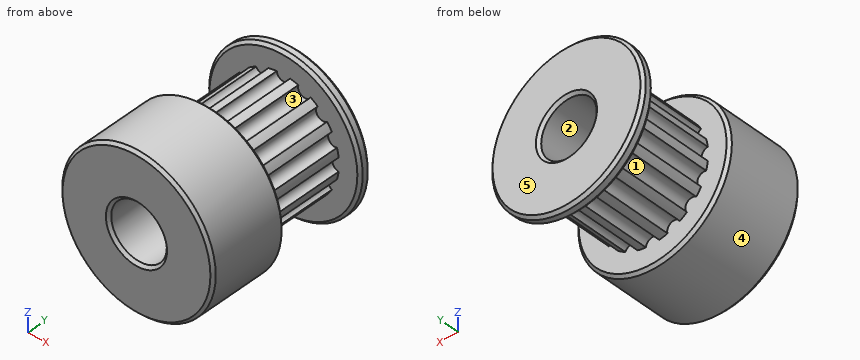
from build123d import *

# Parameters (mm, degrees)
F0_R     = 6.9
F1_DEPTH = 1
F2_R     = 5
F3_DEPTH = 7.5
F4_R     = 6.9
F5_DEPTH = 7
F6_R     = 0.6
F7_DEPTH = 7.5
F8_R     = 2.5
F9_DEPTH = 15.501
F10_SIZE = 0.25


with BuildPart() as f1:
    # F0 (on Front) → F1 (new body)
    with BuildSketch(Plane.XZ):
        Circle(F0_R)
    extrude(amount=F1_DEPTH)

    # F2 (on face) → F3 (join)
    with BuildSketch(Plane.XZ.offset(1)):
        Circle(F2_R)
    extrude(amount=F3_DEPTH)

    # F4 (on face) → F5 (join)
    with BuildSketch(Plane.XZ.offset(8.5)):
        Circle(F4_R)
    extrude(amount=F5_DEPTH)

    # F6 (on face) → F7 (cut, through all)
    with BuildSketch(Plane.XZ.offset(1)):
        with Locations((0, 5)):
            Circle(F6_R)
        with Locations((-1.913417, 4.619398)):
            Circle(F6_R)
        with Locations((-3.535534, 3.535534)):
            Circle(F6_R)
        with Locations((-4.619398, 1.913417)):
            Circle(F6_R)
        with Locations((-5, 0)):
            Circle(F6_R)
        with Locations((-4.619398, -1.913417)):
            Circle(F6_R)
        with Locations((-3.535534, -3.535534)):
            Circle(F6_R)
        with Locations((-1.913417, -4.619398)):
            Circle(F6_R)
        with Locations((0, -5)):
            Circle(F6_R)
        with Locations((1.913417, -4.619398)):
            Circle(F6_R)
        with Locations((3.535534, -3.535534)):
            Circle(F6_R)
        with Locations((4.619398, -1.913417)):
            Circle(F6_R)
        with Locations((5, 0)):
            Circle(F6_R)
        with Locations((4.619398, 1.913417)):
            Circle(F6_R)
        with Locations((3.535534, 3.535534)):
            Circle(F6_R)
        with Locations((1.913417, 4.619398)):
            Circle(F6_R)
    extrude(amount=F7_DEPTH, mode=Mode.SUBTRACT)

    # F8 (on face) → F9 (cut, through all)
    with BuildSketch(Plane.XZ.offset(15.5)):
        Circle(F8_R)
    extrude(amount=-F9_DEPTH, mode=Mode.SUBTRACT)

    # F10
    f10_edges = [f1.edges().sort_by_distance(p)[0] for p in [
        (6.9, -12, 0),
        (-6.9, -8.5, 0),
        (-6.9, -15.5, 0),
        (6.9, -0.5, 0),
        (-6.9, 0, 0),
        (-6.9, -1, 0),
        (-2.5, -15.5, 0),
        (2.5, -7.75, 0),
        (-2.5, 0, 0),
    ]]
    chamfer(f10_edges, length=F10_SIZE)


solid = f1.part
Verification items for the finished model (mm, model axes). Face numbers are marked on the shaded views. A direction names the side the tool comes from. Coordinates: 2 decimals unless noted, no trailing zeros. Loops run counter-clockwise (first coordinate to the right, second up) from the corner with the lowest first, then second, coordinate; pieces in that order, holes last. Notation, with made-up numbers: (36.25, -35) -> (93.25, -35) arc R24 cw to (93.25, -23) -> close; hole circle Ø9 at (69.5, 23). An arc over 180 degrees is marked (long way). Answer as CSV lines item,"result".
1) Depth check by flat-ended pin: pin 1 (5 mm diameter, centred on y = -12.5, z = -4, fed in from -X) (3 decimals); pin 2 (1.5 mm diameter, centred on y = -6.5, z = 5, fed in from -X); pin 3 (1.5 mm diameter, centred on x = 3.5, y = -4, fed in from +Z). Enter the tip coordinate at first touch or a pass-through.
Found:
pin 1,"stops at x = -6.735"
pin 2,"stops at x = -2.63"
pin 3,"stops at z = 4.18"
2) Cross-section at C-C, the plane z = 0. Record the cut outline in (x, y), then the cut area to 3 significant figures.
Found:
outline,"(-6.9, -15.25) -> (-6.65, -15.5) -> (-2.75, -15.5) -> (-2.5, -15.25) -> (-2.5, -0.25) -> (-2.75, 0) -> (-6.65, 0) -> (-6.9, -0.25) -> (-6.9, -0.75) -> (-6.65, -1) -> (-4.4, -1) -> (-4.4, -8.5) -> (-6.65, -8.5) -> (-6.9, -8.75) -> close; (2.5, -15.25) -> (2.75, -15.5) -> (6.65, -15.5) -> (6.9, -15.25) -> (6.9, -8.75) -> (6.65, -8.5) -> (4.4, -8.5) -> (4.4, -1) -> (6.65, -1) -> (6.9, -0.75) -> (6.9, -0.25) -> (6.65, 0) -> (2.75, 0) -> (2.5, -0.25) -> close"
area,"98.5 mm2"
3) Cross-section at A-A, the plane x = 0. Record the cut outline in (y, z).
Found:
outline,"(-15.5, -6.65) -> (-15.25, -6.9) -> (-8.75, -6.9) -> (-8.5, -6.65) -> (-8.5, -4.4) -> (-1, -4.4) -> (-1, -6.65) -> (-0.75, -6.9) -> (-0.25, -6.9) -> (0, -6.65) -> (0, -2.75) -> (-0.25, -2.5) -> (-15.25, -2.5) -> (-15.5, -2.75) -> close; (-15.5, 2.75) -> (-15.25, 2.5) -> (-0.25, 2.5) -> (0, 2.75) -> (0, 6.65) -> (-0.25, 6.9) -> (-0.75, 6.9) -> (-1, 6.65) -> (-1, 4.4) -> (-8.5, 4.4) -> (-8.5, 6.65) -> (-8.75, 6.9) -> (-15.25, 6.9) -> (-15.5, 6.65) -> close"
4) Cross-section at D-D, the plane y = -14.25. Record the cut outline in (x, z).
Found:
outline,"circle Ø13.8 at (0, 0); hole circle Ø5 at (0, 0)"
5) Tool access check on the marked faces 1 and 2. Record the directions out of +Z, -Z, +X, -X, +Y, -Y that give a thin tool (end or side, any length) a straight path to the whole face; none if there is none.
Found:
face 1,"none"
face 2,"+Y, -Y"
6) Thickness scan on L1, parallel to Y at x = 3, z = -4.25; L2, parallel to Z at x = 0, y = -7; L3, parallel to Z at x = -3, y = -3.25. Record the ranges inside material, lowest first. Write a range as from..to.
Found:
L1,"y = -15.5..-8.5, -1..0"
L2,"z = -4.4..-2.5, 2.5..4.4"
L3,"z = -4..-3.81, -3.26..3.26, 3.81..4"
7) Release check for a two-part mould opening along Z. For the marked faces 3, 4 and 5 record: +Z half, -Z half, draft (parallel to the pull), parting line (faces both ways), or undercut.
Found:
face 3,"undercut"
face 4,"parting line"
face 5,"draft"
